Build history of the part. All positions in model axes, mm. A direction names the side the tool comes from. Give positions to 0.01 mm unless a question says otherwise; leave off trailing zeros. Order: outer loops, then holes, each group sorted by start corner. A loop starts at its lowest first (then second) coordinate and runs counter-clockwise, first axis right, second up. Notation, with made-up numbers: (83, 13) - (135, 13) arc R15 ccw to (135, 23) - close; hole circle Ø1 at (55, -4). An arc over 180 degrees is marked (long way). Use a Markdown table: item, result. Add a question column.
(1) Slice it at C-C (x = 7). Write the cut outline in (y, z).
(2) Slice it at A-A (z = 0). Write the cut outline in (x, y), then the cut area to 3 significant figures.
(3) Mould opens along Z. For faces 6 (the face through (2, 22, 5)), 7 (the face through (-9.75, 23.01, -0.07)), 8 (the face through (-9, 23, 7)) say: +Z half, -Z half, draft (parallel to the pull), parting line (faces both ways), or undercut.
(4) Slice it at D-D (z = 8.15). Write the cut outline in (x, y).
(5) Flat gauge pins, fed straight in: pin 1 (8 mm diameter, centred on x = 8.5, z = 9.5, fed in from -Y); pin 2 (5 mm diameter, centred on y = 21, z = -6.5, fed in from -X); pin 3 (2.5 mm diameter, centred on x = 0, z = 6.5, fed in from -Y); pin 4 (6 mm diameter, centred on y = 14, z = 1.5, fed in from +X). Where does each tip first touch, or does it go through?
(6) Wall check: line 1 (Z direction, x = 0, y = 23.4); line 2 (Y direction, x = 4.25, z = -5.5); line 3 (Y direction, x = -1.25, z = -6). Give the ranges that are in metal, low to high.
(7) Which spindle directions (+Z, -Z, +X, -X, +Y, -Y) get a long thin tool onto all of the face, cutting with end or side? Do faces 1 (the face through (-7.5, 3, 0)), 2 (the face through (-0.35, 23.01, -6.59)), 3 (the face through (7.5, 3, 0)), 4 (the face through (2, 6, -6)), 5 (the face through (1.5, 1, 8)). Say none if no direction does.
(8) Slice it at B-B (x = 0). Write the cut outline in (y, z), then the cut area to 3 significant figures.
from build123d import *

# Parameters (mm, degrees)
EXTRUDE_1_DEPTH     = 6
CUT_EXTRUDE_1_DEPTH = 2
SKETCH_4_R          = 5
EXTRUDE_2_DEPTH     = 16
CUT_EXTRUDE_3_REACH = 24
SKETCH_7_R          = 3.1
FILLET_1_R          = 1
SKETCH_8_R          = 11.4
EXTRUDE_3_DEPTH     = 2
SKETCH_9_R          = 3.1
CUT_EXTRUDE_4_DEPTH = 2
SKETCH_10_R         = 1.6
CUT_EXTRUDE_5_DEPTH = 2


with BuildPart() as part:
    # 草图1 → 凸台-拉伸1 (new body)
    with BuildSketch(Plane(origin=(0, 0, 0), x_dir=(1, 0, 0), z_dir=(0, 1, 0))):
        with BuildLine():
            Line((-7.5, 10.372559954), (-7.5, -10.372559954))
            ThreePointArc((-7.5, -10.372559954), (0, -12.8), (7.5, -10.372559954))
            Line((7.5, -10.372559954), (7.5, 10.372559954))
            ThreePointArc((7.5, 10.372559954), (0, 12.8), (-7.5, 10.372559954))
        make_face()
    extrude(amount=EXTRUDE_1_DEPTH)

    # 草图2 → 切除-拉伸1 (cut)
    with BuildSketch(Plane.XZ):
        with BuildLine():
            Line((-1.5, 12.711805537), (-1.5, -12.711805537))
            ThreePointArc((-1.5, -12.711805537), (0, -12.8), (1.5, -12.711805537))
            Line((1.5, -12.711805537), (1.5, 12.711805537))
            ThreePointArc((1.5, 12.711805537), (0, 12.8), (-1.5, 12.711805537))
        make_face()
    extrude(amount=-CUT_EXTRUDE_1_DEPTH, mode=Mode.SUBTRACT)

    # 草图4 → 凸台-拉伸2 (add)
    with BuildSketch(Plane(origin=(0, 6, 0), x_dir=(1, 0, 0), z_dir=(0, 1, 0))):
        Circle(SKETCH_4_R)
    extrude(amount=EXTRUDE_2_DEPTH)

    # 草图7 → 切除-拉伸3 (cut, up to next)
    with BuildSketch(Plane.XZ, mode=Mode.PRIVATE) as cut_extrude_3_sk1:
        Circle(SKETCH_7_R)
    cut_extrude_3_tool1 = extrude(cut_extrude_3_sk1.sketch, amount=-CUT_EXTRUDE_3_REACH, mode=Mode.PRIVATE) & part.part
    add(cut_extrude_3_tool1.solids().sort_by_distance((0, 0, 0))[0], mode=Mode.SUBTRACT)

    # 圆角1
    fillet_1_edges = [part.edges().sort_by_distance(p)[0] for p in [
        (-5, 6, 0),
    ]]
    fillet(fillet_1_edges, radius=FILLET_1_R)

    # 草图8 → 凸台-拉伸3 (add)
    with BuildSketch(Plane(origin=(0, 22, 0), x_dir=(1, 0, 0), z_dir=(0, 1, 0))):
        Circle(SKETCH_8_R)
    extrude(amount=EXTRUDE_3_DEPTH)

    # 草图9 → 切除-拉伸4 (cut)
    with BuildSketch(Plane.XZ.offset(-22)):
        Circle(SKETCH_9_R)
    extrude(amount=-CUT_EXTRUDE_4_DEPTH, mode=Mode.SUBTRACT)

    # 草图10 → 切除-拉伸5 (cut)
    with BuildSketch(Plane(origin=(0, 24, 0), x_dir=(1, 0, 0), z_dir=(0, 1, 0))):
        with Locations((0, 8.15)):
            Circle(SKETCH_10_R)
        with Locations((0, -8.15)):
            Circle(SKETCH_10_R)
        with Locations((-8.15, 0)):
            Circle(SKETCH_10_R)
        with Locations((8.15, 0)):
            Circle(SKETCH_10_R)
    extrude(amount=-CUT_EXTRUDE_5_DEPTH, mode=Mode.SUBTRACT)


solid = part.part
Solution:
| question | item | result |
|---|---|---|
| 1 | outline | (0, -10.72) - (6, -10.72) - (6, 10.72) - (0, 10.72) - close; (22, -9) - (24, -9) - (24, -1.11) - (22, -1.11) - close; (22, 1.11) - (24, 1.11) - (24, 9) - (22, 9) - close |
| 2 | outline | (-11.4, 22) - (-9.75, 22) - (-9.75, 24) - (-11.4, 24) - close; (-7.5, 0) - (-3.1, 0) - (-3.1, 24) - (-6.55, 24) - (-6.55, 22) - (-5, 22) - (-5, 7) arc R1 cw to (-6, 6) - (-7.5, 6) - close; (3.1, 0) - (7.5, 0) - (7.5, 6) - (6, 6) arc R1 cw to (5, 7) - (5, 22) - (6.55, 22) - (6.55, 24) - (3.1, 24) - close; (9.75, 22) - (11.4, 22) - (11.4, 24) - (9.75, 24) - close |
| 2 | area | 134 mm2 |
| 3 | face 6 | draft |
| 3 | face 7 | undercut |
| 3 | face 8 | parting line |
| 4 | outline | (-7.97, 22) - (-1.6, 22) - (-1.6, 24) - (-7.97, 24) - close; (-7.5, 0) - (-1.5, 0) - (-1.5, 2) - (1.5, 2) - (1.5, 0) - (7.5, 0) - (7.5, 6) - (-7.5, 6) - close; (1.6, 22) - (7.97, 22) - (7.97, 24) - (1.6, 24) - close |
| 5 | pin 1 | y = 0 |
| 5 | pin 2 | x = -10.59 |
| 5 | pin 3 | y = 2 |
| 5 | pin 4 | x = 5 |
| 6 | line 1 | -11.4 to -9.75, -6.55 to -3.1, 3.1 to 6.55, 9.75 to 11.4 |
| 6 | line 2 | 0 to 6, 22 to 24 |
| 6 | line 3 | 2 to 6, 22 to 24 |
| 7 | face 1 | +Z, -Z, -X, -Y |
| 7 | face 2 | +Y |
| 7 | face 3 | +Z, -Z, +X, -Y |
| 7 | face 4 | none |
| 7 | face 5 | +Z, -Z, -Y |
| 8 | outline | (2, -12.8) - (6, -12.8) - (6, -6) arc R1 cw to (7, -5) - (22, -5) - (22, -6.55) - (24, -6.55) - (24, -3.1) - (2, -3.1) - close; (2, 3.1) - (24, 3.1) - (24, 6.55) - (22, 6.55) - (22, 5) - (7, 5) arc R1 cw to (6, 6) - (6, 12.8) - (2, 12.8) - close; (22, -11.4) - (24, -11.4) - (24, -9.75) - (22, -9.75) - close; (22, 9.75) - (24, 9.75) - (24, 11.4) - (22, 11.4) - close |
| 8 | area | 159 mm2 |
